Build history of the part. All positions in model axes, mm. Give positions to 0.01 mm unless a question says otherwise; leave off trailing zeros. Write each loop counter-clockwise with the first axis right and the second up, starting at its lowest first coordinate (ties: lowest second). Pieces come first, ordered by that corner, then holes. Notation, with made-up numbers: (-36.75, 50.25) -> (13.25, 50.25) arc R10 cw to (13.25, 65.25) -> close; hole circle Ø11 at (-3, -22.5). An arc over 180 degrees is marked (long way). Write item = value, one per line. Start each with the question number.
Q1. Wall check: line 1 (X direction, y = 70, z = 0.35); line 2 (Y direction, x = -93, z = 2.65); line 3 (X direction, y = 47.5, z = 2.9). Give the ranges that are in metal, low to high.
Q2. Drop flat-ended pins along their axis: P1, Ø2, axis at x = -467.5, z = 2.5, coming from the -Y side; P2, Ø2, axis at y = 71, z = 2, coming from the -X side; P3, Ø2, axis at x = -210, z = 3, coming from the +Y side. Give the stop position or say it passes through.
Q3. Saw through at A-A, the plane x = -319. List the corners of the cut face in (y, z).
Autodesk Inventor part; units mm, degrees
ref_plane "Work Plane2" through (-220, 69, 4) normal (1, 0, 0) x (0, 0, -1)
ref_plane "YZ Plane" through (0, 0, 0) normal (1, 0, 0) x (0, 1, 0)
ref_plane "XZ Plane" through (0, 0, 0) normal (0, 1, 0) x (-1, 0, 0)
sketch "Sketch1" plane through (0, 0, 0) normal (0, 0, 1) x (1, 0, 0)
  line L0 (29, 29) -> (9, 29)
  line L1 (9, 29) -> (9, 25)
  line L2 (9, 25) -> (-31, 25)
  line L3 (-31, 25) -> (-31, 29)
  line L4 (-31, 29) -> (-130.3333, 29)
  line L5 (-130.3333, 29) -> (-130.3333, 25)
  line L6 (-130.3333, 25) -> (-170.3333, 25)
  line L7 (-170.3333, 25) -> (-170.3333, 29)
  line L8 (-170.3333, 29) -> (-269.6667, 29)
  line L9 (-269.6667, 29) -> (-269.6667, 25)
  line L10 (-269.6667, 25) -> (-309.6667, 25)
  line L11 (-309.6667, 25) -> (-309.6667, 29)
  line L12 (-309.6667, 29) -> (-409, 29)
  line L13 (-409, 29) -> (-409, 25)
  line L14 (-409, 25) -> (-449, 25)
  line L15 (-449, 25) -> (-449, 29)
  line L16 (-449, 29) -> (-469, 29)
  line L17 (29, 29) -> (29, 69)
  line L18 (-469, 29) -> (-469, 69)
  line L19 (-469, 49) -> (-556.7501, 49)
  line L20 (9, 69) -> (9, 73)
  line L21 (9, 73) -> (-31, 73)
  line L22 (-31, 73) -> (-31, 69)
  line L23 (-130.3333, 69) -> (-130.3333, 73)
  line L24 (-130.3333, 73) -> (-170.3333, 73)
  line L25 (-409, 73) -> (-449, 73)
  line L26 (-449, 73) -> (-449, 69)
  line L27 (-409, 69) -> (-409, 73)
  line L28 (-309.6667, 73) -> (-309.6667, 69)
  line L29 (-170.3333, 73) -> (-170.3333, 69)
  line L30 (-269.6667, 69) -> (-269.6667, 73)
  line L31 (-269.6667, 73) -> (-309.6667, 73)
  line L32 (-170.3333, 69) -> (-269.6667, 69)
  line L33 (29, 69) -> (9, 69)
  line L34 (-31, 69) -> (-130.3333, 69)
  line L35 (-309.6667, 69) -> (-409, 69)
  line L36 (-449, 69) -> (-469, 69)
  point P0 (0, 0)
  dimension "d0" = 40
  dimension "d1" = 40
  dimension "d2" = 40
  dimension "d3" = 40
  dimension "d4" = 40
  dimension "d5" = 498
  dimension "d6" = 40
extrude "Extrusion1" add sketch "Sketch1" along normal blind 4
sketch "Sketch3" plane through (0, 0, 4) normal (0, 0, 1) x (1, 0, 0)
  line L0 (9, 25) -> (9, 29)
  line L1 (9, 29) -> (29, 29)
  line L2 (29, 29) -> (29, 69)
  line L3 (29, 69) -> (9, 69)
  line L4 (9, 69) -> (9, 73)
  line L5 (9, 73) -> (-31, 73)
  line L6 (-31, 73) -> (-31, 69)
  line L7 (-31, 69) -> (-130.3333, 69)
  line L8 (-130.3333, 69) -> (-130.3333, 73)
  line L9 (-130.3333, 73) -> (-170.3333, 73)
  line L10 (-170.3333, 73) -> (-170.3333, 69)
  line L11 (-170.3333, 69) -> (-269.6667, 69)
  line L12 (-269.6667, 69) -> (-269.6667, 73)
  line L13 (-269.6667, 73) -> (-309.6667, 73)
  line L14 (-309.6667, 73) -> (-309.6667, 69)
  line L15 (-309.6667, 69) -> (-409, 69)
  line L16 (-409, 69) -> (-409, 73)
  line L17 (-409, 73) -> (-449, 73)
  line L18 (-449, 73) -> (-449, 69)
  line L19 (-449, 69) -> (-469, 69)
  line L20 (-469, 69) -> (-469, 29)
  line L21 (-469, 29) -> (-449, 29)
  line L22 (-449, 29) -> (-449, 25)
  line L23 (-449, 25) -> (-409, 25)
  line L24 (-409, 25) -> (-409, 29)
  line L25 (-409, 29) -> (-309.6667, 29)
  line L26 (-309.6667, 29) -> (-309.6667, 25)
  line L27 (-309.6667, 25) -> (-269.6667, 25)
  line L28 (-269.6667, 25) -> (-269.6667, 29)
  line L29 (-269.6667, 29) -> (-170.3333, 29)
  line L30 (-170.3333, 29) -> (-170.3333, 25)
  line L31 (-170.3333, 25) -> (-130.3333, 25)
  line L32 (-130.3333, 25) -> (-130.3333, 29)
  line L33 (-130.3333, 29) -> (-31, 29)
  line L34 (-31, 29) -> (-31, 25)
  line L35 (-31, 25) -> (9, 25)
  line L36 (-234.0151, 149.1478) -> (-234.0151, 116.0125)
  line L37 (25, 54) -> (29, 54)
  line L38 (29, 54) -> (29, 44)
  line L39 (29, 44) -> (25, 44)
  line L40 (25, 44) -> (25, 54)
  point P0 (0, 0)
  point P1 (29, 49)
  dimension "d15" = 498
  dimension "d16" = 4
  dimension "d17" = 10
extrude "Extrusion3" cut sketch "Sketch3" against normal blind 4 contours L39 L40 L37 L2
ref_plane "Work Plane2" through (-220, 69, 4) normal (1, 0, 0) x (0, 0, -1)
mirror "Mirror1" about plane through (-220, 69, 4) normal (1, 0, 0) of "Extrusion3"
properties part number "F1"
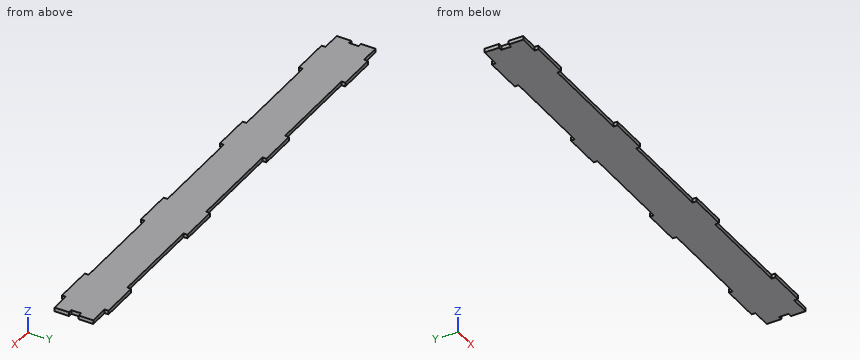
Report:
q1.line_1 = -449 to -409, -309.67 to -269.67, -170.33 to -130.33, -31 to 9
q1.line_2 = 29 to 69
q1.line_3 = -465 to 25
q2.P1 = 29
q2.P2 = -449
q2.P3 = 69
q3.outline = (29, 0) -> (69, 0) -> (69, 4) -> (29, 4) -> close
